Can you work these out from the model? Positions are in its coordinate system, mm. Give positions to 0.01 mm unless a question says otherwise; leave off trailing zeros. Write each loop counter-clockwise with the first axis right and the second up, starting at its lowest first coordinate (ties: lowest second). Pieces come first, ordered by that corner, then holes.
from build123d import *

# Parameters (mm, degrees)
BOSS_EXTRUDE1_DEPTH = 2
BOSS_EXTRUDE2_DEPTH = 2


with BuildPart() as part:
    # Sketch1 → Boss-Extrude1 (new body)
    with BuildSketch(Plane(origin=(0, 0, 0), x_dir=(1, 0, 0), z_dir=(0, 1, 0))):
        with BuildLine():
            Line((14.494481709, 20), (-14.494481709, 20))
            ThreePointArc((-14.494481709, 20), (0, -24.7), (14.494481709, 20))
        make_face()
    extrude(amount=BOSS_EXTRUDE1_DEPTH)

    # Sketch2 → Boss-Extrude2 (add)
    with BuildSketch(Plane(origin=(0, 2, 0), x_dir=(1, 0, 0), z_dir=(0, 1, 0))):
        with BuildLine():
            Line((1, 17.87204521), (1, 19.87485849))
            ThreePointArc((1, 19.87485849), (0, 19.9), (-1, 19.87485849))
            Line((-1, 19.87485849), (-1, 17.87204521))
            ThreePointArc((-1, 17.87204521), (0, 17.9), (1, 17.87204521))
        make_face()
        with BuildLine():
            Line((17.87204521, -1), (19.87485849, -1))
            ThreePointArc((19.87485849, -1), (19.9, 0), (19.87485849, 1))
            Line((19.87485849, 1), (17.87204521, 1))
            ThreePointArc((17.87204521, 1), (17.9, 0), (17.87204521, -1))
        make_face()
        with BuildLine():
            Line((-17.87204521, -1), (-19.87485849, -1))
            ThreePointArc((-19.87485849, -1), (-19.9, 0), (-19.87485849, 1))
            Line((-19.87485849, 1), (-17.87204521, 1))
            ThreePointArc((-17.87204521, 1), (-17.9, 0), (-17.87204521, -1))
        make_face()
        with BuildLine():
            Line((-1, -17.87204521), (-1, -19.87485849))
            ThreePointArc((-1, -19.87485849), (0, -19.9), (1, -19.87485849))
            Line((1, -19.87485849), (1, -17.87204521))
            ThreePointArc((1, -17.87204521), (0, -17.9), (-1, -17.87204521))
        make_face()
    extrude(amount=BOSS_EXTRUDE2_DEPTH)


solid = part.part
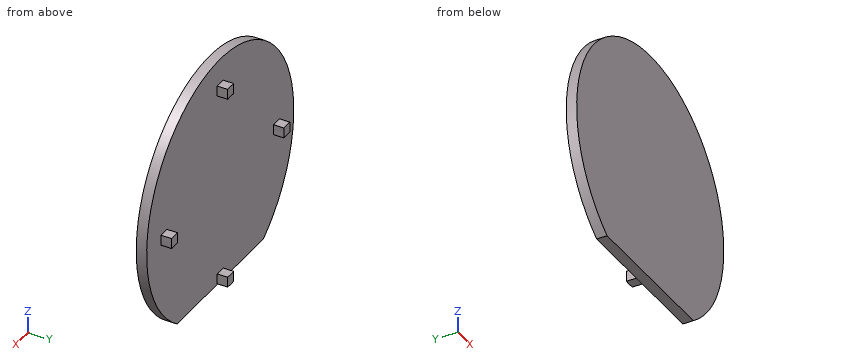
(1) Imagine slicing it at B-B, the plane z = 0. Write out the boundary of the cut face in (x, y).
Returned:
outline: (-24.7, 0) - (24.7, 0) - (24.7, 2) - (19.9, 2) - (19.9, 4) - (17.9, 4) - (17.9, 2) - (-17.9, 2) - (-17.9, 4) - (-19.9, 4) - (-19.9, 2) - (-24.7, 2) - close
(2) If I drill on L1, parallel to Y at x = -18.5, z = 5.5; L2, parallel to X at y = 1.8, z = 0.5; L3, parallel to X at y = 1.65, z = -14.5, over which ranges is the centre line in solid material (lowest first)?
Returned:
L1: y = 0 to 2
L2: x = -24.69 to 24.69
L3: x = -20 to 20
(3) Imagine slicing it at A-A, the plane x = 0. Write out the boundary of the cut face in (y, z), plus the area to 3 significant figures.
Returned:
outline: (0, -20) - (2, -20) - (2, -19.9) - (4, -19.9) - (4, -17.9) - (2, -17.9) - (2, 17.9) - (4, 17.9) - (4, 19.9) - (2, 19.9) - (2, 24.7) - (0, 24.7) - close
area: 97.4 mm2
(4) Imagine slicing it at D-D, the plane x = 17. Write out the boundary of the cut face in (y, z), plus the area to 3 significant figures.
Returned:
outline: (0, -17.92) - (2, -17.92) - (2, 17.92) - (0, 17.92) - close
area: 71.7 mm2
(5) Imagine slicing it at C-C, the plane y = 0.95. Write out the boundary of the cut face in (x, z).
Returned:
outline: (-14.49, -20) - (14.49, -20) arc R24.7 ccw (long way) to start
(6) Will these pins go through, and if not, where does the flat tip stop? P1, Ø2, axis at y = 2.5, z = 19, coming from the +X side; P2, Ø1, axis at x = 12, y = 3, coming from the -Z side; P3, Ø0.6, axis at x = 18.5, y = 3.5, coming from the -Z side; P4, Ø2, axis at y = 2.5, z = -19.5, coming from the +X side.
Returned:
P1: stops at x = 16.77
P2: passes through
P3: stops at z = -1
P4: stops at x = 16.21
